```python
from build123d import *

# Parameters (mm, degrees)
SKETCH_W     = 16
SKETCH_H     = 38
SKETCH_R     = 1.6
PAD_DEPTH    = 3
SKETCH002_R  = 1.6
PAD001_DEPTH = 3


with BuildPart() as part:
    # Sketch → Pad (new body)
    with BuildSketch(Plane.XY):
        with Locations((2, 5)):
            Rectangle(SKETCH_W, SKETCH_H)
        Circle(SKETCH_R, mode=Mode.SUBTRACT)
        with Locations((0, 20)):
            Circle(SKETCH_R, mode=Mode.SUBTRACT)
    extrude(amount=PAD_DEPTH)

    # Sketch002 → Pad001 (join)
    with BuildSketch(Plane.XY.offset(3)):
        Polygon((-15, -14), (-15, 4), (-8.477261, 4), (-8.477261, 24), (10, 24), (10, -14), align=None)
        with Locations((0, 20)):
            Circle(SKETCH002_R, mode=Mode.SUBTRACT)
        Circle(SKETCH002_R, mode=Mode.SUBTRACT)
        with Locations((-11.917612, 0)):
            Circle(SKETCH002_R, mode=Mode.SUBTRACT)
        with Locations((-11.917612, -10)):
            Circle(SKETCH002_R, mode=Mode.SUBTRACT)
    extrude(amount=PAD001_DEPTH)


solid = part.part
```
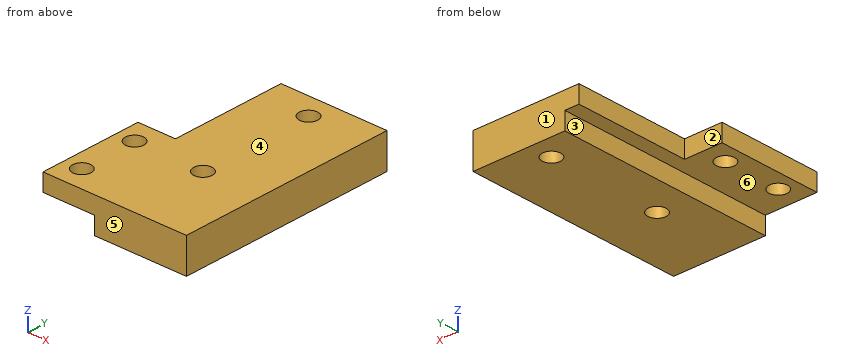
Source: CAD feature listing. Evaluate the final solid. Frame: model axes, mm. Face numbers are marked on the shaded views. A direction names the side the tool comes from. Give positions to 0.01 mm unless a question says otherwise; leave off trailing zeros. Order: outer loops, then holes, each group sorted by start corner. A loop starts at its lowest first (then second) coordinate and runs counter-clockwise, first axis right, second up.
(1) Material intervals for line 1 along Y through (x, z) = (0, 4); line 2 along X through (y, z) = (15, 4.55); line 3 along Y through (x, z) = (-1.25, 4.7), sorted ascending.
(2) Contact query for flat-ended pins moving along their axis: P1, Ø5, axis at x = -11.92, y = 0, coming from the +Z side; P2, Ø4, axis at x = -11.92, y = -10, coming from the -Z side; P3, Ø3.5, axis at x = -10.5, z = 5, coming from the +Y side; P4, Ø3.5, axis at y = 13.5, z = 2, coming from the -X side. Output: stop coordinate, or through.
(3) Pull-direction query (Z, two-part tool) for the marked faces 4, 5 and 6; classes: +Z half, -Z half, draft (parallel to the pull), parting line (faces both ways), or undercut.
(4) Section query C-C (z = 4.55). Return the cut outline in (x, y), plus the area to 3 significant figures.
(5) Section query B-B (x = -0.5). Return the cut outline in (y, z).
(6) Access query for the marked faces 1, 2 and 3. Directions: +Z, -Z, +X, -X, +Y, -Y. A direction counts if a zero-diameter tool reaches every point of the face in a straight line with its end or side. Return the directions, or none.
(7) Section query A-A (y = -10). Return the cut outline in (x, z).
(8) Section query D-D (y = 0). Return the cut outline in (x, z), plus the area to 3 significant figures.
Outcome:
1. line 1: y = -14 to -1.6, 1.6 to 18.4, 21.6 to 24
1. line 2: x = -8.48 to 10
1. line 3: y = -14 to -1, 1 to 19, 21 to 24
2. P1: stops at z = 6
2. P2: stops at z = 3
2. P3: stops at y = 4
2. P4: stops at x = -8.48
3. face 4: +Z half
3. face 5: draft
3. face 6: -Z half
4. outline: (-15, -14) - (10, -14) - (10, 24) - (-8.48, 24) - (-8.48, 4) - (-15, 4) - close; hole circle Ø3.2 at (-11.92, -10); hole circle Ø3.2 at (-11.92, 0); hole circle Ø3.2 at (0, 0); hole circle Ø3.2 at (0, 20)
4. area: 787 mm2
5. outline: (-14, 0) - (-1.52, 0) - (-1.52, 6) - (-14, 6) - close; (1.52, 0) - (18.48, 0) - (18.48, 6) - (1.52, 6) - close; (21.52, 0) - (24, 0) - (24, 6) - (21.52, 6) - close
6. face 1: +Z, -Z, +X, -X, +Y
6. face 2: +Z, -Z, -X, +Y
6. face 3: -Z, -X, +Y, -Y
7. outline: (-15, 3) - (-13.52, 3) - (-13.52, 6) - (-15, 6) - close; (-10.32, 3) - (-6, 3) - (-6, 0) - (10, 0) - (10, 6) - (-10.32, 6) - close
8. outline: (-15, 3) - (-13.52, 3) - (-13.52, 6) - (-15, 6) - close; (-10.32, 3) - (-6, 3) - (-6, 0) - (-1.6, 0) - (-1.6, 6) - (-10.32, 6) - close; (1.6, 0) - (10, 0) - (10, 6) - (1.6, 6) - close
8. area: 94.2 mm2
